Autodesk Inventor part; units mm, degrees
ref_plane "YZ Plane" through (0, 0, 0) normal (1, 0, 0) x (0, 1, 0)
ref_plane "XZ Plane" through (0, 0, 0) normal (0, 1, 0) x (-1, 0, 0)
ref_plane "XY Plane" through (0, 0, 0) normal (0, 0, 1) x (1, 0, 0)
sketch "Sketch1" plane through (0, 0, 0) normal (0, 0, 1) x (1, 0, 0)
  line L0 (-12.1708, 16.0073) -> (13.2292, 16.0073)
  line L1 (13.2292, 16.0073) -> (13.2292, -34.7927)
  line L2 (13.2292, -34.7927) -> (-12.1708, -34.7927)
  line L3 (-12.1708, -34.7927) -> (-12.1708, 16.0073)
  line L4 (11.9592, 14.7373) -> (-10.9008, 14.7373)
  line L5 (-10.9008, 14.7373) -> (-10.9008, -33.5227)
  line L6 (-10.9008, -33.5227) -> (11.9592, -33.5227)
  line L7 (11.9592, -33.5227) -> (11.9592, 14.7373)
  point P0 (0, 0)
  dimension "d0" = 25.4
  dimension "d1" = 50.8
  dimension "d2" = 1.27
extrude "Extrusion1" add sketch "Sketch1" along normal blind 769.62
sketch "Sketch2" plane through (-12.1708, 16.0073, 0) normal (0, 1, 0) x (1, 0, 0)
  circle A0 centre (12.7, -12.7) radius 1.7272
  line L0 (25.4, 0) -> (0, 0)
  line L1 (0, 0) -> (0, -769.62)
  point P0 (12.1708, 0)
  dimension "d5" = 3.4544
  dimension "d6" = 12.7
  dimension "d7" = 12.7
extrude "Extrusion2" cut sketch "Sketch2" against normal through all
pattern_linear "Rectangular Pattern1" count 77 spacing 25.4 along (0, 0, 1) of "Extrusion2"
sketch "Sketch5" plane through (-12.1708, -34.7927, 0) normal (-1, 0, 0) x (0, 0, 1)
  circle A0 centre (44.45, 25.4) radius 2.3813
  circle A1 centre (44.45, 38.1) radius 2.3813
  circle A2 centre (44.45, 12.7) radius 2.3813
  line L0 (44.45, 12.7) -> (44.45, 38.1)
  line L1 (0, 0) -> (769.62, 0)
  line L2 (0, 50.8) -> (0, 0)
  point P0 (0, 34.7927)
  dimension "d43" = 25.4
  dimension "d44" = 4.7625
  dimension "d45" = 25.4
  dimension "d46" = 44.45
extrude "Extrusion5" cut sketch "Sketch5" against normal through all
equation "\"d3\" = d13"
equation "\"d10\" = d14"
equation "\"d13\" = 769.62"
equation "\"d14\" = d13"
properties part number "Long bar 32.3 - VersaFrame"
The listing builds one solid part. Answer for the finished solid, in the listing's coordinates (mm). A direction names the side the tool comes from. Give positions to 0.01 mm unless a question says otherwise; leave off trailing zeros. Loops run counter-clockwise (first coordinate to the right, second up) from the corner with the lowest first, then second, coordinate; pieces in that order, holes last.
Item 1: A cutting plane is placed at B-B (z = 71.5). Give the vertices of the cut face in (x, y).
Derived:
outline: (-12.17, -34.79) - (13.23, -34.79) - (13.23, 16.01) - (-12.17, 16.01) - close; hole (-10.9, -33.52) - (11.96, -33.52) - (11.96, 14.74) - (-10.9, 14.74) - close
Item 2: A cutting plane is placed at A-A (x = -5.25). Give the vertices of the cut face in (y, z).
Derived:
outline: (-34.79, 0) - (-33.52, 0) - (-33.52, 769.62) - (-34.79, 769.62) - close; (14.74, 0) - (16.01, 0) - (16.01, 769.62) - (14.74, 769.62) - close
Item 3: A tool of negligible diameter and unlimited length cuts with its end or side. For faces 5 (the flat face through (-10.901, -9, 379)), 6 (the flat face through (13.229, -9, 379)), from which of +Z, -Z, +X, -X, +Y, -Y can it reach the whole face along a straight path? Write none if from no direction.
Derived:
face 5: +Z, -Z
face 6: +Z, -Z, +X, +Y, -Y
Item 4: Determine the mould class of faces 1 (the flat face through (11.959, -10, 379)), 2 (the flat face through (1, -34.793, 379)), 3 (the flat face through (-12.171, -10, 379)), 4 (the flat face through (0, -33.523, 379)) for opening direction X: +X half, -X half, draft (parallel to the pull), parting line (faces both ways), or undercut.
Derived:
face 1: undercut
face 2: draft
face 3: -X half
face 4: undercut
Item 5: Find the intervals of material crossed by line 1 along X through (y, z) = (4.5, 527); line 2 along Y through (x, z) = (4.5, 498.5); line 3 along Y through (x, z) = (12.2, 44.45), in increasing order.
Derived:
line 1: x = -12.17 to -10.9, 11.96 to 13.23
line 2: y = -34.79 to -33.52, 14.74 to 16.01
line 3: y = -34.79 to -24.47, -19.71 to -11.77, -7.01 to 0.93, 5.69 to 16.01
Item 6: This flat-tipped pin is pushed along its axis until it touches: pin 1 Ø3 at (x, z) = (0.53, 63.5) entering from -Y. Where does it stop, or does it pass through?
Derived:
pin 1: passes through
